Drawing for the job (mm, zero at the part's lowest x, y, z). A direction names the side the tool comes from. Round coordinates to 2 decimals unless told otherwise and drop trailing zeros. Write each loop counter-clockwise with the first axis right and the second up, starting at its lowest first coordinate (ties: lowest second). Pieces come first, ordered by that corner, then holes. Notation, with made-up numbers: (67, 25.25) -> (115, 25.25) arc R34 cw to (115, 55.25) -> close; hole circle Ø8 at (78.5, 47). An arc over 180 degrees is marked (long way). Answer in a Markdown table with one row per item. Add a question column.
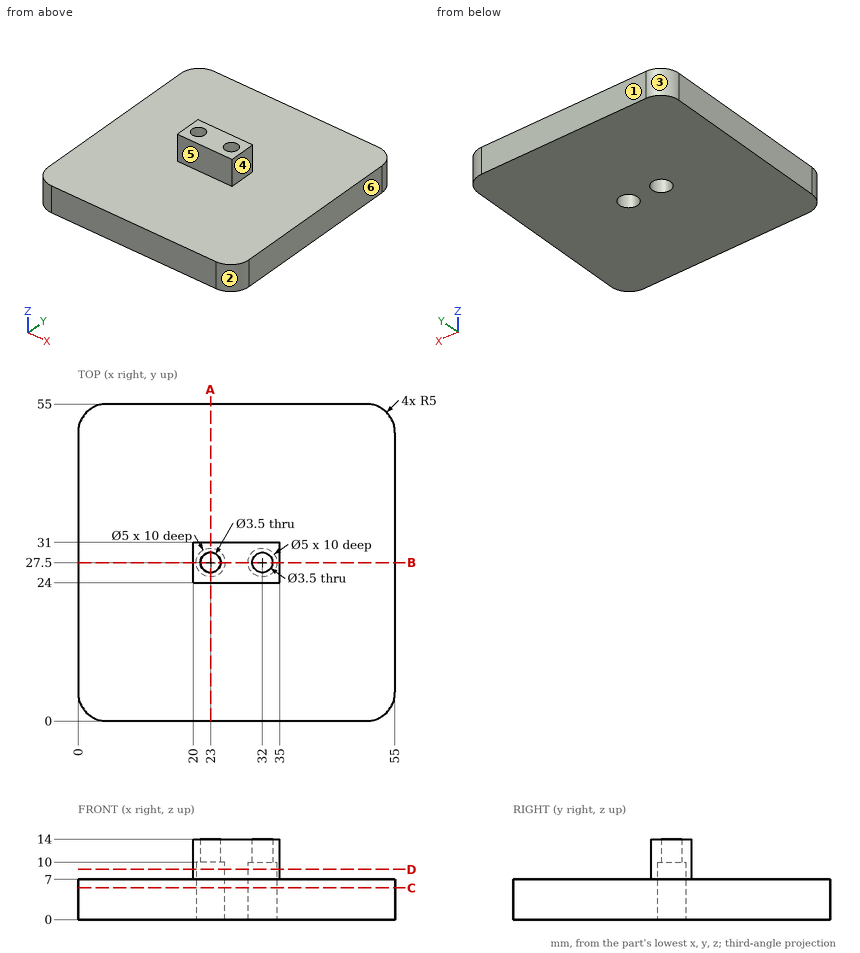
(1) Saw through at A-A (x = 23). List the corners of the cut face in (y, z).
(2) Mould opens along X. For the marked faces 1, 2 and 3 say: pulls with the +X half, pulls with the -X half, needs draft (parallel to the pull), parting line crosses it, or undercut.
(3) Saw through at D-D (z = 8.75). List the corners of the cut face in (x, y), plus the area to 3 significant figures.
(4) Saw through at C-C (z = 5.5). List the corners of the cut face in (x, y).
(5) Drop flat-ended pins along their axis: P1, Ø2, axis at x = 23, y = 27.5, coming from the -Z side; P2, Ø1, axis at y = 28, z = 9.5, coming from the -X side; P3, Ø6, axis at x = 12, y = 19, coming from the +Z side; P4, Ø1.5, axis at x = 24, y = 28, coming from the -Z side. Give the stop position or say it passes through.
(6) Which spindle directions (+Z, -Z, +X, -X, +Y, -Y) get a long thin tool onto all of the face, cutting with end or side? Do the marked faces 4, 5 and 6. Say none if no direction does.
(7) Saw through at B-B (y = 27.5). List the corners of the cut face in (x, z).
(8) Probe line 1 along Y through (x, z) = (23, 12); line 2 along Z through (x, y) = (43, 44); line 3 along Y through (x, z) = (34, 1). List the from-to ranges inside material, lowest first.
Answer sheet:
| question | item | result |
|---|---|---|
| 1 | outline | (0, 0) -> (25, 0) -> (25, 10) -> (25.75, 10) -> (25.75, 14) -> (24, 14) -> (24, 7) -> (0, 7) -> close; (29.25, 10) -> (30, 10) -> (30, 0) -> (55, 0) -> (55, 7) -> (31, 7) -> (31, 14) -> (29.25, 14) -> close |
| 2 | face 1 | needs draft |
| 2 | face 2 | pulls with the +X half |
| 2 | face 3 | pulls with the -X half |
| 3 | outline | (20, 24) -> (35, 24) -> (35, 31) -> (20, 31) -> close; hole circle Ø5 at (23, 27.5); hole circle Ø5 at (32, 27.5) |
| 3 | area | 65.7 mm² |
| 4 | outline | (0, 5) arc R5 ccw to (5, 0) -> (50, 0) arc R5 ccw to (55, 5) -> (55, 50) arc R5 ccw to (50, 55) -> (5, 55) arc R5 ccw to (0, 50) -> close; hole circle Ø5 at (23, 27.5); hole circle Ø5 at (32, 27.5) |
| 5 | P1 | passes through |
| 5 | P2 | stops at x = 20 |
| 5 | P3 | stops at z = 7 |
| 5 | P4 | stops at z = 10 |
| 6 | face 4 | +Z, +X, +Y, -Y |
| 6 | face 5 | +Z, +X, -X, -Y |
| 6 | face 6 | +Z, -Z, +X, +Y, -Y |
| 7 | outline | (0, 0) -> (20.5, 0) -> (20.5, 10) -> (21.25, 10) -> (21.25, 14) -> (20, 14) -> (20, 7) -> (0, 7) -> close; (24.75, 10) -> (25.5, 10) -> (25.5, 0) -> (29.5, 0) -> (29.5, 10) -> (30.25, 10) -> (30.25, 14) -> (24.75, 14) -> close; (33.75, 10) -> (34.5, 10) -> (34.5, 0) -> (55, 0) -> (55, 7) -> (35, 7) -> (35, 14) -> (33.75, 14) -> close |
| 8 | line 1 | y = 24 to 25.75, 29.25 to 31 |
| 8 | line 2 | z = 0 to 7 |
| 8 | line 3 | y = 0 to 26, 29 to 55 |
